from build123d import *

# Parameters (mm, degrees)
CYLINDER_R        = 2.5
CYLINDER_DEPTH    = 70
CYLINDER001_R     = 2.5
CYLINDER001_DEPTH = 70
BOX004_W          = 68.15
BOX004_H          = 15
BOX004_DEPTH      = 50
BOX008_W          = 30
BOX008_H          = 100
BOX008_DEPTH      = 70
EXTRUDE003_DEPTH  = 25
BOX006_W          = 40
BOX006_H          = 120
BOX006_DEPTH      = 60
TUBE_R            = 45
TUBE_R_2          = 19.07
TUBE_DEPTH        = 50
BOX001_W          = 82
BOX001_H          = 58
BOX001_DEPTH      = 44.4
BOX007_W          = 5
BOX007_H          = 5
BOX007_DEPTH      = 44.4
SKETCH001_R       = 5
EXTRUDE001_DEPTH  = 4
EXTRUDE002_DEPTH  = 15
SKETCH_R          = 12.3
EXTRUDE_DEPTH     = 5
BOX_W             = 75.7
BOX_H             = 45
BOX_DEPTH         = 44.4
BOX002_W          = 175
BOX002_H          = 90
BOX002_DEPTH      = 50
BOX005_W          = 68.15
BOX005_H          = 15
BOX005_DEPTH      = 50


with BuildPart() as throughholecylinder2:
    # Cylinder → Cylinder (new body)
    with BuildSketch(Plane(origin=(-86, -18, -20), x_dir=(1, 0, 0), z_dir=(0, 0, 1))):
        Circle(CYLINDER_R)
    extrude(amount=CYLINDER_DEPTH)


with BuildPart() as throughholecylinder1:
    # Cylinder001 → Cylinder001 (new body)
    with BuildSketch(Plane(origin=(-86, 56, -20), x_dir=(1, 0, 0), z_dir=(0, 0, 1))):
        Circle(CYLINDER001_R)
    extrude(amount=CYLINDER001_DEPTH)


with BuildPart() as cube004:
    # Box004 → Box004 (new body)
    with BuildSketch(Plane(origin=(41, -26, -10), x_dir=(1, 0, 0), z_dir=(0, 0, 1))):
        with Locations((34.075, 7.5)):
            Rectangle(BOX004_W, BOX004_H)
    extrude(amount=BOX004_DEPTH)


with BuildPart() as steeringshaftcutter:
    # Box008 → Box008 (new body)
    with BuildSketch(Plane(origin=(136, -31, -14), x_dir=(1, 0, 0), z_dir=(0, 0, 1))):
        with Locations((15, 50)):
            Rectangle(BOX008_W, BOX008_H)
    extrude(amount=BOX008_DEPTH)


with BuildPart() as fingers:
    # Sketch004 (on Face2 of Tube) → Extrude003 (new body)
    with BuildSketch(Plane(origin=(120.15, 19, 40), x_dir=(1, 0, 0), z_dir=(0, 0, 1))):
        with BuildLine():
            Line((16.519435, -9.5375), (20.849562, -12.0375))
            ThreePointArc((12.0375, -20.849562), (17.023596, -17.023596), (20.849562, -12.0375))
            Line((12.0375, -20.849562), (9.5375, -16.519435))
            ThreePointArc((9.5375, -16.519435), (13.488062, -13.488062), (16.519435, -9.5375))
        make_face()
        with BuildLine():
            Line((0, -24.075), (0, -19.07))
            ThreePointArc((-9.535, -16.515104), (-4.935679, -18.420206), (0, -19.07))
            Line((-9.535, -16.515104), (-12.0375, -20.849562))
            ThreePointArc((-12.0375, -20.849562), (-6.231069, -23.254664), (0, -24.075))
        make_face()
        with BuildLine():
            Line((-20.849562, -12.0375), (-16.515104, -9.535))
            ThreePointArc((-19.07, 0), (-18.420206, -4.935679), (-16.515104, -9.535))
            Line((-19.07, 0), (-24.075, 0))
            ThreePointArc((-24.075, 0), (-23.254664, -6.231069), (-20.849562, -12.0375))
        make_face()
        with BuildLine():
            Line((-16.519435, 9.5375), (-20.849562, 12.0375))
            ThreePointArc((-12.0375, 20.849562), (-17.023596, 17.023596), (-20.849562, 12.0375))
            Line((-12.0375, 20.849562), (-9.5375, 16.519435))
            ThreePointArc((-9.5375, 16.519435), (-13.488062, 13.488062), (-16.519435, 9.5375))
        make_face()
        with BuildLine():
            Line((0, 24.075), (0, 19.075))
            ThreePointArc((9.5375, 16.519435), (4.936973, 18.425035), (0, 19.075))
            Line((9.5375, 16.519435), (12.0375, 20.849562))
            ThreePointArc((12.0375, 20.849562), (6.231069, 23.254664), (0, 24.075))
        make_face()
        with BuildLine():
            Line((16.515104, 9.535), (20.849562, 12.0375))
            ThreePointArc((24.075, 0), (23.254664, 6.231069), (20.849562, 12.0375))
            Line((19.07, 0), (24.075, 0))
            ThreePointArc((19.07, 0), (18.420206, 4.935679), (16.515104, 9.535))
        make_face()
    extrude(amount=EXTRUDE003_DEPTH)


with BuildPart() as fingers_1:
    # Extrude003 placement: moved
    add(fingers.part.moved(Location((0, 0, -5))))


with BuildPart() as obj1:
    # Box006 → Box006 (new body)
    with BuildSketch(Plane(origin=(55, -34, -17), x_dir=(1, 0, 0), z_dir=(0, 0, 1))):
        with Locations((20, 60)):
            Rectangle(BOX006_W, BOX006_H)
    extrude(amount=BOX006_DEPTH)


with BuildPart() as steeringshaftcutdown:
    # Tube → Tube (new body)
    with BuildSketch(Plane(origin=(120.15, 19, -10), x_dir=(1, 0, 0), z_dir=(0, 0, 1))):
        Circle(TUBE_R)
        Circle(TUBE_R_2, mode=Mode.SUBTRACT)
    extrude(amount=TUBE_DEPTH)

    # Cut001: cut obj1
    add(obj1.part, mode=Mode.SUBTRACT)

    # Fusion004: union Fingers
    add(fingers_1.part)


with BuildPart() as steeringshaftcutdown_1:
    # Fusion004 placement: moved
    add(steeringshaftcutdown.part.moved(Location((-12, 0, 0))))

    # Cut002: cut SteeringShaftCutter
    add(steeringshaftcutter.part, mode=Mode.SUBTRACT)


with BuildPart() as motorhead:
    # Box001 → Box001 (new body)
    with BuildSketch(Plane(origin=(-82, -9.63, 0), x_dir=(1, 0, 0), z_dir=(0, 0, 1))):
        with Locations((41, 29)):
            Rectangle(BOX001_W, BOX001_H)
    extrude(amount=BOX001_DEPTH)


with BuildPart() as obj2:
    # Box007 → Box007 (new body)
    with BuildSketch(Plane(origin=(75.7, 16.87, 0), x_dir=(1, 0, 0), z_dir=(0, 0, 1))):
        with Locations((2.5, 2.5)):
            Rectangle(BOX007_W, BOX007_H)
    extrude(amount=BOX007_DEPTH)


with BuildPart() as obj3:
    # Sketch001 (on Face3 of Extrude) → Extrude001 (new body)
    with BuildSketch(Plane.XY.offset(49.4)):
        with Locations((-58.7, 20.37)):
            Circle(SKETCH001_R)
    extrude(amount=EXTRUDE001_DEPTH)


with BuildPart() as obj4:
    # Sketch002 (on Face3 of Extrude001) → Extrude002 (new body)
    with BuildSketch(Plane.XY.offset(53.4)):
        with BuildLine():
            Line((-62.7, 23.37), (-62.7, 17.37))
            ThreePointArc((-62.7, 17.37), (-53.7, 20.37), (-62.7, 23.37))
        make_face()
    extrude(amount=EXTRUDE002_DEPTH)


with BuildPart() as motorshaftassembly:
    # Sketch (on Face6 of Box001) → Extrude (new body)
    with BuildSketch(Plane(origin=(-82, -9.63, 44.4), x_dir=(1, 0, 0), z_dir=(0, 0, 1))):
        with Locations((23.3, 30)):
            Circle(SKETCH_R)
    extrude(amount=EXTRUDE_DEPTH)

    # Fusion: union obj3, obj4
    add(obj3.part)
    add(obj4.part)


with BuildPart() as motor:
    # Box → Box (new body)
    with BuildSketch(Plane(origin=(0, -3.13, 0), x_dir=(1, 0, 0), z_dir=(0, 0, 1))):
        with Locations((37.85, 22.5)):
            Rectangle(BOX_W, BOX_H)
    extrude(amount=BOX_DEPTH)

    # Fusion005: union MotorHead, obj2, MotorShaftAssembly
    add(motorhead.part)
    add(obj2.part)
    add(motorshaftassembly.part)


with BuildPart() as steeringshaftmotormount:
    # Box002 → Box002 (new body)
    with BuildSketch(Plane(origin=(-92, -26, -10), x_dir=(1, 0, 0), z_dir=(0, 0, 1))):
        with Locations((87.5, 45)):
            Rectangle(BOX002_W, BOX002_H)
    extrude(amount=BOX002_DEPTH)

    # Cut: cut Motor
    add(motor.part, mode=Mode.SUBTRACT)

    # Fusion006: union SteeringShaftCutDown
    add(steeringshaftcutdown_1.part)


with BuildPart() as cut004:
    # Box005 → Box005 (new body)
    with BuildSketch(Plane(origin=(41, 49, -10), x_dir=(1, 0, 0), z_dir=(0, 0, 1))):
        with Locations((34.075, 7.5)):
            Rectangle(BOX005_W, BOX005_H)
    extrude(amount=BOX005_DEPTH)

    # Fusion007: union Cube004, SteeringShaftMotorMount
    add(cube004.part)
    add(steeringshaftmotormount.part)

    # Cut003: cut ThroughHoleCylinder1
    add(throughholecylinder1.part, mode=Mode.SUBTRACT)

    # Cut004: cut ThroughHoleCylinder2
    add(throughholecylinder2.part, mode=Mode.SUBTRACT)


solid = cut004.part
Design review of the part built by this model. Coordinates are the model's own, in mm. A direction names the side the tool comes from. Give positions to 0.01 mm unless a question says otherwise; leave off trailing zeros. Order: outer loops, then holes, each group sorted by start corner. A loop starts at its lowest first (then second) coordinate and runs counter-clockwise, first axis right, second up.
1. Add section B-B, the plane x = -86. State the section outline as (y, z) points.
Solution:
outline: (-26, -10) - (-20.5, -10) - (-20.5, 40) - (-26, 40) - close; (-15.5, -10) - (53.5, -10) - (53.5, 40) - (-15.5, 40) - close; (58.5, -10) - (64, -10) - (64, 40) - (58.5, 40) - close
2. Add section A-A, the plane z = 48. State how many separate pieces and enclosed holes the cut face has, then the cut area to 3 significant figures.
Solution:
separate pieces: 6
enclosed holes: 0
area: 339 mm2
3. For pin 1 Ø4.5 at (x, y) = (-86, 56) entering from -Z; pin 2 Ø2.5 at (y, z) = (-4, 51) entering from +X; pin 3 Ø17.5 at (x, y) = (9.5, 19) entering from +Z, all flat-tipped, find the tip position at first contact; note any pin that passes through.
Solution:
pin 1: passes through
pin 2: stops at x = 108.15
pin 3: stops at z = 0
4. Mouldability with a two-part tool opening along Y and no side actions: class faces 4 (the flat face through (0, 45, 20)), 5 (the flat face through (114, 40, 60)), 6 (the cylindrical face through (123.17, -23.42, 14.65)), 7 (the flat face through (97.381, 0.348, 49.86)) as +Y half, -Y half, draft (parallel to the pull), parting line (faces both ways), or undercut.
Solution:
face 4: undercut
face 5: draft
face 6: -Y half
face 7: undercut
5. To check wall thickness, follow L1, parallel to X at y = 19, z = 18; L2, parallel to Y at x = -86, z = 25; L3, parallel to Y at x = 0.5, z = 22. State the ranges of each line that lie inside material, in increasing order.
Solution:
L1: x = -92 to -82, 80.7 to 89.08, 127.22 to 136
L2: y = -26 to -20.5, -15.5 to 53.5, 58.5 to 64
L3: y = -26 to -3.13, 41.87 to 64
6. Tool access review of faces 1 (the cylindrical face through (94.711, 32.537, 49.86)), 2 (the flat face through (-42, 48.37, 20)), 3 (the flat face through (126.804, 8.23, 49.86)): name each direction out of +Z, -Z, +X, -X, +Y, -Y from which nothing blocks a thin tool from reaching the whole face with its end or side.
Solution:
face 1: +Z, -Z
face 2: +Z
face 3: +Z, +X
7. Add section C-C, the plane x = -22.5. State the section outline as (y, z) points, then the cut area to 3 significant figures.
Solution:
outline: (-26, -10) - (64, -10) - (64, 40) - (48.37, 40) - (48.37, 0) - (-9.63, 0) - (-9.63, 40) - (-26, 40) - close
area: 2,180 mm2
8. Add section D-D, the plane y = 51. State the section outline as (x, z) points, then the cut area to 3 significant figures.
Solution:
outline: (-92, -10) - (136, -10) - (136, 40) - (-92, 40) - close
area: 11,400 mm2
